Verification items for the finished model (mm, model axes). Face numbers are marked on the shaded views. Give positions to 0.01 mm unless a question says otherwise; leave off trailing zeros. Write each loop counter-clockwise with the first axis right and the second up, starting at its lowest first coordinate (ties: lowest second). Pieces come first, ordered by that corner, then holes.
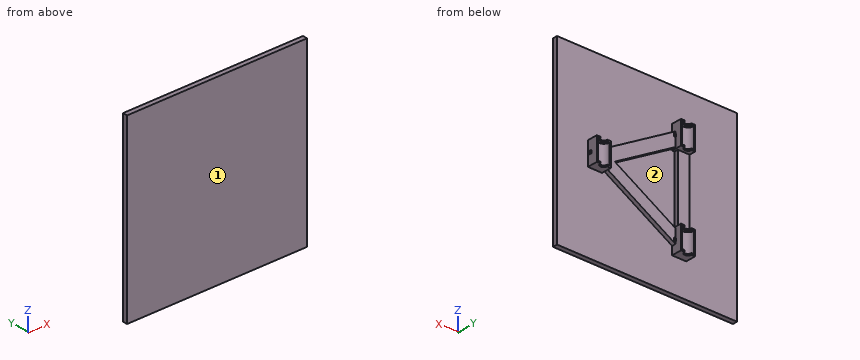
from build123d import *

# Parameters (mm, degrees)
BOTTOM_W                     = 230
BOTTOM_H                     = 230
BOSS_EXTRUDE2_DEPTH          = 6
TRIANGLE_DEPTH               = 5
BOSS_EXTRUDE4_DEPTH          = 8
BOSS_EXTRUDE4_DEPTH_BACK     = 6
SKETCH5_W                    = 18
SKETCH5_H                    = 29.5
ROD_CUTOUT_REACH             = 209.436
SKETCH6_R                    = 4.5
ROD_CUTOUT_DIRECTION_2_REACH = 209.436
LM8SOCKET_START              = -2
SKETCH7_R                    = 7.5
LM8SOCKET_1_DEPTH            = 25.5
LM8SOCKET_START_2            = -27.5
SKETCH8_R                    = 7.5
LM8SOCKET_2_DEPTH            = 25.5
SKETCH9_R                    = 4.5
CUT_EXTRUDE4_DEPTH           = 29.5
CUT_EXTRUDE5_START           = -2
SKETCH11_R                   = 7.5
CUT_EXTRUDE5_DEPTH           = 25.5
SKETCH12_W                   = 4
SKETCH12_H                   = 2.5
CUT_EXTRUDE8_DEPTH           = 20
FILLET1_R                    = 1
FILLET2_R                    = 1
SKETCH13_W                   = 4
SKETCH13_H                   = 2.5
CUT_EXTRUDE9_DEPTH           = 20


with BuildPart() as part:
    # bottom → Boss-Extrude2 (new body)
    with BuildSketch(Plane(origin=(0, 0, 0), x_dir=(1, 0, 0), z_dir=(0, 1, 0))):
        with Locations((-18.058375635, -12.779187817)):
            Rectangle(BOTTOM_W, BOTTOM_H)
    extrude(amount=BOSS_EXTRUDE2_DEPTH)

    # Sketch4 → Triangle (add)
    with BuildSketch(Plane(origin=(0, 6, 0), x_dir=(1, 0, 0), z_dir=(0, 1, 0))):
        Polygon((-68.058375635, 59.720812183), (-68.058375635, -85.279187817), (57.515307914, -12.779187817), align=None)
        Polygon((-53.058375635, -59.298425704), (-53.058375635, 33.740050069), (27.515307914, -12.779187817), align=None, mode=Mode.SUBTRACT)
    extrude(amount=TRIANGLE_DEPTH)

    # Sketch5 → Boss-Extrude4 (add, two sides: drawn at the far end of the back side and taken through both)
    with BuildSketch(Plane(origin=(0, 11, 0), x_dir=(1, 0, 0), z_dir=(0, 1, 0)).offset(-BOSS_EXTRUDE4_DEPTH_BACK)):
        with Locations((-59.058375635, 44.970812183)):
            Rectangle(SKETCH5_W, SKETCH5_H)
        with Locations((-59.058375635, -70.529187817)):
            Rectangle(SKETCH5_W, SKETCH5_H)
        with Locations((48.515307914, -12.779187817)):
            Rectangle(SKETCH5_W, SKETCH5_H)
    extrude(amount=BOSS_EXTRUDE4_DEPTH + BOSS_EXTRUDE4_DEPTH_BACK)

    # Rod cutout: up to this face of the body (flat: up to its plane)
    rod_cutout_end = Plane(part.part.faces().sort_by_distance((-59.058375635, 12.5, -59.720812183))[0])
    # Sketch6 → Rod cutout (cut, up to the picked face)
    with BuildSketch(Plane.XY.offset(-30.220812183), mode=Mode.PRIVATE) as rod_cutout_sk1:
        with Locations((-59.058375635, 19)):
            Circle(SKETCH6_R)
    rod_cutout_tool1 = split(extrude(rod_cutout_sk1.sketch, amount=-ROD_CUTOUT_REACH, mode=Mode.PRIVATE), bisect_by=rod_cutout_end, keep=Keep.BOTH, mode=Mode.PRIVATE)
    add(rod_cutout_tool1.solids().sort_by(Axis((-59.058376, 19, -30.220812), (0, 0, -1)))[0], mode=Mode.SUBTRACT)

    # Rod cutout direction 2: up to this face of the body (flat: up to its plane)
    rod_cutout_direction_2_end = Plane(part.part.faces().sort_by_distance((-59.058375635, 12.5, 85.279187817))[0])
    # Sketch6 → Rod cutout direction 2 (cut, up to the picked face)
    with BuildSketch(Plane.XY.offset(-30.220812183), mode=Mode.PRIVATE) as rod_cutout_direction_2_sk1:
        with Locations((-59.058375635, 19)):
            Circle(SKETCH6_R)
    rod_cutout_direction_2_tool1 = split(extrude(rod_cutout_direction_2_sk1.sketch, amount=ROD_CUTOUT_DIRECTION_2_REACH, mode=Mode.PRIVATE), bisect_by=rod_cutout_direction_2_end, keep=Keep.BOTH, mode=Mode.PRIVATE)
    add(rod_cutout_direction_2_tool1.solids().sort_by(Axis((-59.058376, 19, -30.220812), (0, 0, 1)))[0], mode=Mode.SUBTRACT)

    # Sketch7 → LM8Socket 1 (cut)
    with BuildSketch(Plane.XY.offset(-30.220812183).offset(LM8SOCKET_START)):
        with Locations((-59.058375635, 19)):
            Circle(SKETCH7_R)
    extrude(amount=-LM8SOCKET_1_DEPTH, mode=Mode.SUBTRACT)

    # Sketch8 → LM8Socket 2 (cut)
    with BuildSketch(Plane(origin=(0, 0, 55.779187817), x_dir=(-1, 0, 0), z_dir=(0, 0, -1)).offset(LM8SOCKET_START_2)):
        with Locations((59.058375635, 19)):
            Circle(SKETCH8_R)
    extrude(amount=LM8SOCKET_2_DEPTH, mode=Mode.SUBTRACT)

    # Sketch9 → Cut-Extrude4 (cut)
    with BuildSketch(Plane(origin=(0, 0, -1.970812183), x_dir=(-1, 0, 0), z_dir=(0, 0, -1))):
        with Locations((-48.515307914, 19)):
            Circle(SKETCH9_R)
    extrude(amount=-CUT_EXTRUDE4_DEPTH, mode=Mode.SUBTRACT)

    # Sketch11 → Cut-Extrude5 (cut)
    with BuildSketch(Plane(origin=(0, 0, -1.970812183), x_dir=(-1, 0, 0), z_dir=(0, 0, -1)).offset(CUT_EXTRUDE5_START)):
        with Locations((-48.515307914, 19)):
            Circle(SKETCH11_R)
    extrude(amount=-CUT_EXTRUDE5_DEPTH, mode=Mode.SUBTRACT)

    # Sketch12 → Cut-Extrude8 (cut)
    with BuildSketch(Plane.ZY.offset(68.058375635)):
        with Locations((-44.970812183, 9.75)):
            Rectangle(SKETCH12_W, SKETCH12_H)
        with Locations((70.529187817, 9.75)):
            Rectangle(SKETCH12_W, SKETCH12_H)
    extrude(amount=-CUT_EXTRUDE8_DEPTH, mode=Mode.SUBTRACT)

    # Fillet1
    fillet1_edges = [part.edges().sort_by_distance(p)[0] for p in [
        (-50.058375635, 11, -44.970812183),
    ]]
    fillet(fillet1_edges, radius=FILLET1_R)

    # Fillet2
    fillet2_edges = [part.edges().sort_by_distance(p)[0] for p in [
        (-50.058375635, 11, 70.529187817),
    ]]
    fillet(fillet2_edges, radius=FILLET2_R)

    # Sketch13 → Cut-Extrude9 (cut)
    with BuildSketch(Plane(origin=(57.515307914, 0, 0), x_dir=(0, 0, -1), z_dir=(1, 0, 0))):
        with Locations((-12.779187817, 9.75)):
            Rectangle(SKETCH13_W, SKETCH13_H)
    extrude(amount=-CUT_EXTRUDE9_DEPTH, mode=Mode.SUBTRACT)


solid = part.part
Item 1: Sectioned sample at D-D on x = 32. Record the cut outline in (y, z).
Answer key:
outline: (0, -102.22) - (6, -102.22) - (6, -1.95) - (11, -1.95) - (11, 27.51) - (6, 27.51) - (6, 127.78) - (0, 127.78) - close
Item 2: Sectioned sample at A-A on x = 68.5. Record the cut outline in (y, z), then the cut area to 3 significant figures.
Answer key:
outline: (0, -102.22) - (6, -102.22) - (6, 127.78) - (0, 127.78) - close
area: 1,380 mm2
Item 3: Scan lines: line 1 along Y through (x, z) = (71, -85); line 2 along X through (y, z) = (9, 29); line 3 along X through (y, z) = (12.25, 68). Record each from-to range of solid material in increasing order.
Answer key:
line 1: y = 0 to 6
line 2: x = -68.06 to -53.06, -0.58 to 29.42
line 3: x = -68.06 to -62.33, -55.79 to -50.06
Item 4: Depth check by flat-ended pin: pin 1 (3 mm diameter, centred on x = -61, y = 11, fed in from -Z); pin 2 (10 mm diameter, centred on y = 12, z = 28, fed in from -X); pin 3 (4.5 mm diameter, centred on x = -59, z = 5.5, fed in from +Y). Enter the tip coordinate at first touch or a pass-through.
Answer key:
pin 1: stops at z = -59.72
pin 2: stops at x = -68.06
pin 3: stops at y = 11
Item 5: Release check for a two-part mould opening along X. For the marked faces 1 and 2 record: released by +X, released by -X, zero draft, split by the parting line, or undercut.
Answer key:
face 1: zero draft
face 2: undercut
Item 6: Sectioned sample at C-C on x = -8.5. Record the cut outline in (y, z).
Answer key:
outline: (0, -102.22) - (6, -102.22) - (6, -25.33) - (11, -25.33) - (11, -8.01) - (6, -8.01) - (6, 33.57) - (11, 33.57) - (11, 50.89) - (6, 50.89) - (6, 127.78) - (0, 127.78) - close
Item 7: Sectioned sample at B-B on z = -70.5. Record the cut outline in (x, y).
Answer key:
outline: (-133.06, 0) - (96.94, 0) - (96.94, 6) - (-133.06, 6) - close
